Geometry check sheet. Reference: the model listing, model coordinates, mm. A direction names the side the tool comes from. Give positions to 0.01 mm unless a question says otherwise; leave off trailing zeros. Order: outer loops, then holes, each group sorted by start corner. A loop starts at its lowest first (then second) coordinate and runs counter-clockwise, first axis right, second up. Notation, with made-up numbers: (24.25, 11.25) - (80.25, 11.25) arc R23 ccw to (80.25, 28.25) - close; hole circle Ø6 at (50.25, 61.25). An arc over 180 degrees is marked (long way). Put each result on its own line as item: value. Start each with the question number.
```python
from build123d import *

# Parameters (mm, degrees)
BOSS_EXTRUDE1_DEPTH = 7
SKETCH2_W           = 14
SKETCH2_H           = 14
BOSS_EXTRUDE2_DEPTH = 7
SKETCH2_3_W         = 14
SKETCH2_3_H         = 14
BOSS_EXTRUDE3_DEPTH = 14


with BuildPart() as part:
    # Sketch1 → Boss-Extrude1 (new body)
    with BuildSketch(Plane(origin=(0, 0, 0), x_dir=(1, 0, 0), z_dir=(0, 1, 0))):
        with BuildLine():
            Line((0, -7), (0, -14))
            Line((0, -14), (-50, -14))
            Line((-50, -14), (-50, 0))
            Line((-50, 0), (-21, 0))
            ThreePointArc((-21, 0), (-18.949747468, -4.949747468), (-14, -7))
            Line((-14, -7), (0, -7))
        make_face()
    extrude(amount=BOSS_EXTRUDE1_DEPTH)

    # Mirror1: part across plane


with BuildPart() as part_1:
    add(part.part)
    add(part.part.mirror(Plane(origin=(-21, 7, 0), x_dir=(1, 0, 0), z_dir=(0, 0, 1))))

    # Sketch2 → Boss-Extrude2 (add)
    with BuildSketch(Plane(origin=(0, 7, 0), x_dir=(1, 0, 0), z_dir=(0, 1, 0))):
        with Locations((-43, -7)):
            Rectangle(SKETCH2_W, SKETCH2_H)
    extrude(amount=BOSS_EXTRUDE2_DEPTH)

    # Sketch2<3> → Boss-Extrude3 (add)
    with BuildSketch(Plane(origin=(0, 7, 0), x_dir=(1, 0, 0), z_dir=(0, 1, 0))):
        with Locations((-43, 7)):
            Rectangle(SKETCH2_3_W, SKETCH2_3_H)
    extrude(amount=BOSS_EXTRUDE3_DEPTH)


solid = part_1.part
```
Item 1: Release check for a two-part mould opening along Z. For faces 4 (the face through (-31, 6, -14)), 5 (the face through (-7, 3, 7)), 6 (the face through (-50, 8, 0)) record: +Z half, -Z half, draft (parallel to the pull), parting line (faces both ways), or undercut.
Item 2: Cross-section at D-D (x = -43). Enter the section's corners in (y, z), and give its area (3 significant figures).
Item 3: Thickness scan on line 1 along Z through (x, y) = (-42, 19.75); line 2 along Y through (x, z) = (-27, -1.25); line 3 along X through (y, z) = (12.5, -2.25). Record the ranges inside material, lowest first.
Item 4: Cross-section at C-C (z = 11). Enter the section's corners in (x, y).
Item 5: Cross-section at B-B (y = 3). Enter the section's corners in (x, z), and give its area (3 significant figures).
Item 6: Set-up check for faces 1 (the face through (-22, 7, 0)), 2 (the face through (-7, 3, -7)), 3 (the face through (-43, 14, 7)): record each of +Z, -Z, +X, -X, +Y, -Y from which the full face is reachable in a straight line by a thin tool's end or side.
Item 7: Gauge pin test, flat ends, axial feed: pin 1 Ø5 at (x, z) = (-11.5, -6) entering from +Y; pin 2 Ø7 at (x, z) = (-45.5, 7.5) entering from +Y; pin 3 Ø2 at (x, y) = (-45.5, 17) entering from +Z. Record the tip position at first contact, or that the pin passes through.
Item 8: Cross-section at A-A (x = -9.5). Enter the section's corners in (y, z).
Recorded:
1. face 4: -Z half
1. face 5: undercut
1. face 6: draft
2. outline: (0, -14) - (21, -14) - (21, 0) - (14, 0) - (14, 14) - (0, 14) - close
2. area: 490 mm^2
3. line 1: z = -14 to 0
3. line 2: y = 0 to 7
3. line 3: x = -50 to -36
4. outline: (-50, 0) - (0, 0) - (0, 7) - (-36, 7) - (-36, 14) - (-50, 14) - close
5. outline: (-50, -14) - (0, -14) - (0, -7) - (-14, -7) arc R7 cw to (-14, 7) - (0, 7) - (0, 14) - (-50, 14) - close
5. area: 1,130 mm^2
6. face 1: +Z, -Z, +X, +Y
6. face 2: +X, +Y, -Y
6. face 3: +Z, +X, -X, +Y
7. pin 1: stops at y = 7
7. pin 2: stops at y = 14
7. pin 3: stops at z = 0
8. outline: (0, -14) - (7, -14) - (7, -7) - (0, -7) - close; (0, 7) - (7, 7) - (7, 14) - (0, 14) - close
